from build123d import *

# Parameters (mm, degrees)
SKETCH_R             = 7
PAD_DEPTH            = 10
SKETCH001_R          = 7
SKETCH001_R_2        = 5
POCKET_DEPTH         = 7
FILLET_R             = 2
BODY_PLACEMENT_ANGLE = 180


with BuildPart() as part:
    # Sketch → Pad (new body)
    with BuildSketch(Plane.XZ):
        Circle(SKETCH_R)
    extrude(amount=PAD_DEPTH)

    # Sketch001 (on Face3 of Pad) → Pocket (cut)
    with BuildSketch(Plane.XZ.offset(10)):
        Circle(SKETCH001_R)
        Circle(SKETCH001_R_2, mode=Mode.SUBTRACT)
    extrude(amount=-POCKET_DEPTH, mode=Mode.SUBTRACT)

    # Fillet
    fillet_edges = [part.edges().sort_by_distance(p)[0] for p in [
        (-5, -10, 0),
    ]]
    fillet(fillet_edges, radius=FILLET_R)


with BuildPart() as part_1:
    # Body placement: moved
    add(part.part.rotate(Axis((0, 0, 0), (0, 0, 1)), BODY_PLACEMENT_ANGLE))


solid = part_1.part
Could you check a few things on this model? Use its own coordinates, in mm. A direction names the side the tool comes from. Coordinates: 2 decimals unless noted, no trailing zeros. Write each loop counter-clockwise with the first axis right and the second up, starting at its lowest first coordinate (ties: lowest second). Pieces come first, ordered by that corner, then holes. Notation, with made-up numbers: (79, -39.75) - (91, -39.75) arc R18 cw to (91, -15.75) - close; hole circle Ø11 at (-9.5, -7). An arc over 180 degrees is marked (long way). Put each result on its own line as item: value. Start each with the question number.
Q1. I want a section at C-C on y = 1.75. Write out the boundary of the cut face in (x, z).
Q2. I'm going to push flat-ended pins straight in: P1, Ø3, axis at y = 6, z = -1.5, coming from the -X side; P2, Ø1.5, axis at y = 9, z = -2.5, coming from the +X side; P3, Ø3, axis at x = -3, y = 5, coming from the -Z side. Where does each tip first touch, or does it pass through?
Q3. Which directions (+Z, -Z, +X, -X, +Y, -Y) give clear straight access to the entire face, cutting with the end or side of a thin tool? Please do faces 1 (the cylindrical face through (-6.466, 1.479, -2.681)), 2 (the cylindrical face through (1.08, 5.54, -4.88)).
Q4. Please list where these lines run through material, in increasing order: L1, parallel to Z at x = 0, y = 4.5; L2, parallel to Y at x = -4.5, z = 2.75; L3, parallel to Z at x = 4.25, y = 1.25.
Q5. I want a section at B-B on x = 0. Write out the boundary of the cut face in (y, z), plus the area to 3 significant figures.
Q6. I want a section at A-A on z = 0. Write out the boundary of the cut face in (x, y).
Q7. I want a section at D-D on y = 6. Write out the boundary of the cut face in (x, z).
Checks:
1. outline: circle Ø14 at (0, 0)
2. P1: x = -5
2. P2: x = 4.54
2. P3: z = -4.77
3. face 1: +Y, -Y
3. face 2: +Y
4. L1: -5 to 5
4. L2: 0 to 3
4. L3: -5.56 to 5.56
5. outline: (0, -7) - (3, -7) - (3, -5) - (8, -5) arc R2 ccw to (10, -3) - (10, 3) arc R2 ccw to (8, 5) - (3, 5) - (3, 7) - (0, 7) - close
5. area: 110 mm²
6. outline: (-7, 0) - (7, 0) - (7, 3) - (5, 3) - (5, 8) arc R2 ccw to (3, 10) - (-3, 10) arc R2 ccw to (-5, 8) - (-5, 3) - (-7, 3) - close
7. outline: circle Ø10 at (0, 0)
